Design review of the part built by this model. Coordinates are the model's own, in mm. A direction names the side the tool comes from. Coordinates: 2 decimals unless noted, no trailing zeros. Write each loop counter-clockwise with the first axis right and the second up, starting at its lowest first coordinate (ties: lowest second). Pieces come first, ordered by that corner, then holes.
Q1. Add section D-D, the plane y = -57. Give the boundary of the cut face in (x, z).
Q2. Add section C-C, the plane x = -35.5. Give the boundary of the cut face in (y, z), plus the area to 3 significant figures.
Q3. Add section A-A, the plane y = -49.5. Give the boundary of the cut face in (x, z).
Q4. Add section B-B, the plane x = -20.5. Give the boundary of the cut face in (y, z).
Q5. Machinability: for faces 4 (the face through (-41.859, -11.216, 1.479)), 5 (the face through (-9.51, -18.7, 1.48)), 6 (the face through (-73.993, -21.358, 1.479)), 7 (the face through (-90.204, -36.286, 1.479)), which of the approach directions +Z, -Z, +X, -X, +Y, -Y give a long, thin tool a straight path to every point of the face, cutting with its end or side? Answer none if there is none.
Q6. The part is to be moulded in two halves that separate along Y. For faces 1 (the face through (-38, -38, 0)), 2 (the face through (-15.91, -7.37, 1.48)), 3 (the face through (-65.655, -20.698, 1.479)), say which applies: +Y half, -Y half, draft (parallel to the pull), parting line (faces both ways), or undercut.
Q7. To check wall thickness, follow probe 1 along Y at (x, z) = (-20.5, 2.3); probe 2 along Y at (x, z) = (-21, 0.8); probe 3 along Y at (x, z) = (-72, 1.3). State the ranges of each line that lie inside material, in increasing order.
Q8. Clearance check with flat-ended pins moving along their axes: pin 1 Ø1 at (x, z) = (-12, 1.5) entering from -Y; pin 2 Ø3 at (x, y) = (-13, -53) entering from -Z. State where each tip first meets the part, or that it passes through.
from build123d import *

# Parameters (mm, degrees)
SKETCH_1_R      = 2
EXTRUDE_1_DEPTH = 3


with BuildPart() as part:
    # 草图1 → 凸台-拉伸1 (new body)
    with BuildSketch(Plane.XY):
        Polygon((0, 0), (0, -60), (-50, -60), (-50.776457135, -62.897777479), (-53.674234614, -62.121320344), (-52.897777479, -59.223542865), (-98.296291314, -47.059047745), (-96.743377044, -41.263492787), (-93.845599565, -42.039949922), (-92.939732907, -38.65920953), (-89.076029602, -39.694485711), (-89.334848647, -40.660411537), (-86.437071168, -41.436868672), (-86.178252123, -40.470942846), (-80.769067496, -41.920329499), (-79.992610361, -39.02255202), (-85.401794988, -37.573165367), (-85.142975943, -36.607239541), (-88.040753422, -35.830782406), (-88.299572467, -36.796708232), (-92.163275772, -35.761432052), (-91.257409114, -32.38069166), (-94.155186593, -31.604234524), (-92.728879324, -24.84662833), (-74.376288624, -19.929066473), (-73.599831489, -22.826843952), (-70.219091097, -21.920977294), (-69.183814917, -25.784680599), (-70.149740743, -26.043499644), (-69.373283608, -28.941277123), (-68.407357781, -28.682458078), (-66.957971129, -34.091642705), (-64.06019365, -33.31518557), (-65.509580302, -27.906000943), (-64.543654476, -27.647181898), (-65.320111611, -24.749404419), (-66.286037438, -25.008223464), (-67.321313618, -21.144520159), (-63.940573226, -20.238653501), (-64.717030361, -17.340876022), (-18.352590699, -4.917561857), (-17.576133564, -7.815339336), (-14.195393172, -6.909472678), (-13.160116992, -10.773175983), (-14.126042818, -11.031995028), (-13.349585683, -13.929772507), (-12.383659856, -13.670953462), (-10.934273204, -19.080138089), (-8.036495725, -18.303680954), (-9.485882378, -12.894496327), (-8.519956551, -12.635677282), (-9.296413687, -9.737899803), (-10.262339513, -9.996718848), (-11.297615693, -6.133015543), (-7.916875301, -5.227148885), (-8.693332437, -2.329371406), align=None)
        with Locations((-20.5, -49.5)):
            Circle(SKETCH_1_R, mode=Mode.SUBTRACT)
    extrude(amount=EXTRUDE_1_DEPTH)


solid = part.part
Here are the results:
1. outline: (-61.2, 0) - (0, 0) - (0, 3) - (-61.2, 3) - close
2. outline: (-60, 0) - (-9.51, 0) - (-9.51, 3) - (-60, 3) - close
2. area: 151 mm2
3. outline: (-89.19, 0) - (-22.5, 0) - (-22.5, 3) - (-89.19, 3) - close; (-18.5, 0) - (0, 0) - (0, 3) - (-18.5, 3) - close
4. outline: (-60, 0) - (-51.5, 0) - (-51.5, 3) - (-60, 3) - close; (-47.5, 0) - (-5.49, 0) - (-5.49, 3) - (-47.5, 3) - close
5. face 4: +Z, -Z, -X, +Y
5. face 5: +Z, -Z
5. face 6: +Z, -Z, +Y
5. face 7: +Z, -Z, -X
6. face 1: draft
6. face 2: +Y half
6. face 3: undercut
7. probe 1: y = -60 to -51.5, -47.5 to -5.49
7. probe 2: y = -60 to -51.44, -47.56 to -5.63
7. probe 3: y = -54.11 to -22.4
8. pin 1: stops at y = -60
8. pin 2: stops at z = 0
